```python
from build123d import *

# Parameters (mm, degrees)
SKETCH1_R                = 140
SKETCH1_R_2              = 97
BOSS_EXTRUDE1_DEPTH      = 112.5
SKETCH2_R                = 23.5
BOSS_EXTRUDE2_DEPTH      = 32
CIRPATTERN1_COUNT        = 3
MIRROR1_COPY_1_SKETCH_R  = 23.5
MIRROR1_COPY_1_DEPTH     = 32
MIRROR1_COPY_2_SKETCH_R  = 23.5
MIRROR1_COPY_2_DEPTH     = 32
SKETCH3_R                = 28.1
CUT_EXTRUDE1_DEPTH       = 310
BOSS_EXTRUDE3_REACH      = 450.894
BOSS_EXTRUDE3_END_RADIUS = 140
SKETCH4_R                = 100
SKETCH5_R                = 50
CUT_EXTRUDE2_DEPTH       = 25
SKETCH6_R                = 10.15
CUT_EXTRUDE3_DEPTH       = 13
BOSS_EXTRUDE4_REACH      = 400.629
BOSS_EXTRUDE4_END_RADIUS = 140
SKETCH7_R                = 37.5
SKETCH7_R_2              = 28.1
SKETCH8_R                = 37.5
BOSS_EXTRUDE5_DEPTH      = 10


with BuildPart() as part:
    # Sketch1 → Boss-Extrude1 (new, symmetric)
    with BuildSketch(Plane(origin=(0, 0, 0), x_dir=(1, 0, 0), z_dir=(0, 1, 0))):
        with Locations(Location((0, 0, 0), (0, 0, 270))):
            Circle(SKETCH1_R)
        with Locations(Location((0, 0, 0), (0, 0, 270))):
            Circle(SKETCH1_R_2, mode=Mode.SUBTRACT)
    extrude(amount=BOSS_EXTRUDE1_DEPTH, both=True)

    # Sketch2 → Boss-Extrude2 (add)
    with BuildSketch(Plane(origin=(0, 112.5, 0), x_dir=(1, 0, 0), z_dir=(0, 1, 0))):
        with BuildLine():
            ThreePointArc((175, -50), (225, 0), (175, 50))
            Line((175, 50), (130.766968306, 50))
            ThreePointArc((130.766968306, 50), (137.672392953, 25.42267135), (140, 0))
            ThreePointArc((140, 0), (137.672392953, -25.42267135), (130.766968306, -50))
            Line((130.766968306, -50), (175, -50))
        make_face()
        with Locations(Location((175, 0, 0), (0, 0, 270))):
            Circle(SKETCH2_R, mode=Mode.SUBTRACT)
    boss_extrude2 = extrude(amount=-BOSS_EXTRUDE2_DEPTH)

    # CirPattern1: Boss-Extrude2 ×3 about axis
    cirpattern1_axis = Axis((0, 0, 0), (0, 1, 0))
    for i in range(1, CIRPATTERN1_COUNT):
        add(boss_extrude2.rotate(cirpattern1_axis, i * 360 / CIRPATTERN1_COUNT))

    # Mirror1: Boss-Extrude2 across plane
    add(boss_extrude2.mirror(Plane.ZX))

    # Mirror1 copy 1 sketch → Mirror1 copy 1 (add)
    with BuildSketch(Plane(origin=(0, -112.5, 0), x_dir=(-0.4999999999999998, 0, -0.8660254037844387), z_dir=(0, -1, 0))):
        with BuildLine():
            ThreePointArc((175, 50), (225, 0), (175, -50))
            Line((175, -50), (130.766968306, -50))
            ThreePointArc((130.766968306, -50), (137.672392953, -25.42267135), (140, 0))
            ThreePointArc((140, 0), (137.672392953, 25.42267135), (130.766968306, 50))
            Line((130.766968306, 50), (175, 50))
        make_face()
        with Locations((175, 0)):
            Circle(MIRROR1_COPY_1_SKETCH_R, mode=Mode.SUBTRACT)
    extrude(amount=-MIRROR1_COPY_1_DEPTH)

    # Mirror1 copy 2 sketch → Mirror1 copy 2 (add)
    with BuildSketch(Plane(origin=(0, -112.5, 0), x_dir=(-0.5000000000000004, 0, 0.8660254037844384), z_dir=(0, -1, 0))):
        with BuildLine():
            ThreePointArc((175, 50), (225, 0), (175, -50))
            Line((175, -50), (130.766968306, -50))
            ThreePointArc((130.766968306, -50), (137.672392953, -25.42267135), (140, 0))
            ThreePointArc((140, 0), (137.672392953, 25.42267135), (130.766968306, 50))
            Line((130.766968306, 50), (175, 50))
        make_face()
        with Locations((175, 0)):
            Circle(MIRROR1_COPY_2_SKETCH_R, mode=Mode.SUBTRACT)
    extrude(amount=-MIRROR1_COPY_2_DEPTH)

    # Sketch3 → Cut-Extrude1 (cut)
    with BuildSketch(Plane(origin=(-160, 0, 0), x_dir=(0, 0, -1), z_dir=(1, 0, 0))):
        with Locations(Location((0, 0, 0), (0, 0, 180))):
            Circle(SKETCH3_R)
    extrude(amount=CUT_EXTRUDE1_DEPTH, mode=Mode.SUBTRACT)

    # Boss-Extrude3: up to this cylinder (the profile starts outside it)
    boss_extrude3_end = Plane(origin=(0, 0, 0), z_dir=(0, -1, 0)) * Cylinder(BOSS_EXTRUDE3_END_RADIUS, 1182.788, mode=Mode.PRIVATE)
    # Sketch4 → Boss-Extrude3 (add, up to the surface)
    with BuildSketch(Plane(origin=(-160, 0, 0), x_dir=(0, 0, -1), z_dir=(1, 0, 0)), mode=Mode.PRIVATE) as boss_extrude3_sk1:
        with Locations(Location((0, 0, 0), (0, 0, 180))):
            Circle(SKETCH4_R)
    boss_extrude3_tool1 = extrude(boss_extrude3_sk1.sketch, amount=BOSS_EXTRUDE3_REACH, mode=Mode.PRIVATE) - boss_extrude3_end
    add(boss_extrude3_tool1.solids().sort_by_distance((-160, 0, 0))[0])

    # Sketch5 → Cut-Extrude2 (cut)
    with BuildSketch(Plane.ZY.offset(160)):
        Circle(SKETCH5_R)
    extrude(amount=-CUT_EXTRUDE2_DEPTH, mode=Mode.SUBTRACT)

    # Sketch6 → Cut-Extrude3 (cut)
    with BuildSketch(Plane.ZY.offset(160)):
        with Locations((0, 75)):
            Circle(SKETCH6_R)
        with Locations((64.951905284, -37.5)):
            Circle(SKETCH6_R)
        with Locations((-64.951905284, -37.5)):
            Circle(SKETCH6_R)
    extrude(amount=-CUT_EXTRUDE3_DEPTH, mode=Mode.SUBTRACT)

    # Boss-Extrude4: up to this cylinder (the profile starts outside it)
    boss_extrude4_end = Plane(origin=(0, 0, 0), z_dir=(0, -1, 0)) * Cylinder(BOSS_EXTRUDE4_END_RADIUS, 1082.258, mode=Mode.PRIVATE)
    # Sketch7 → Boss-Extrude4 (add, up to the surface)
    with BuildSketch(Plane(origin=(165, 0, 0), x_dir=(0, 0, -1), z_dir=(1, 0, 0)), mode=Mode.PRIVATE) as boss_extrude4_sk1:
        Circle(SKETCH7_R)
        with Locations(Location((0, 0, 0), (0, 0, 180))):
            Circle(SKETCH7_R_2, mode=Mode.SUBTRACT)
    boss_extrude4_tool1 = extrude(boss_extrude4_sk1.sketch, amount=-BOSS_EXTRUDE4_REACH, mode=Mode.PRIVATE) - boss_extrude4_end
    add(boss_extrude4_tool1.solids().sort_by_distance((165, 0, 36.43934))[0])

    # Sketch8 → Boss-Extrude5 (add)
    with BuildSketch(Plane(origin=(165, 0, 0), x_dir=(0, 0, -1), z_dir=(1, 0, 0))):
        Circle(SKETCH8_R)
    extrude(amount=-BOSS_EXTRUDE5_DEPTH)


solid = part.part
```
Read the model definition and answer for the solid it produces. Units are mm, in the model's axes. A direction names the side the tool comes from. Coordinates: 2 decimals unless noted, no trailing zeros. Write each loop counter-clockwise with the first axis right and the second up, starting at its lowest first coordinate (ties: lowest second). Pieces come first, ordered by that corner, then holes. Notation, with made-up numbers: (83, 37.5) -> (124, 37.5) arc R26 ccw to (124, 73.5) -> close; hole circle Ø9 at (31.5, 73.5). An arc over 180 degrees is marked (long way). Answer as a JSON object with one key per item and string values.
Q1. The part is cut by section C-C on x = -87.5. Give the number of separate pieces and of enclosed holes in the cut face, then the cut area to 3 significant figures.
The answers:
{"separate pieces": "6", "enclosed holes": "0", "area": "36,100 mm2"}
Q2. The part is cut by section B-B on y = 75. Give the vertices of the cut face in (x, z).
The answers:
{"outline": "(-160, -66.14) -> (-123.39, -66.14) arc R140 ccw (long way) to (-123.39, 66.14) -> (-160, 66.14) -> (-160, 10.15) -> (-147, 10.15) -> (-147, -10.15) -> (-160, -10.15) -> close; hole circle Ø194 at (0, 0)"}
Q3. A tool of negligible diameter and unlimited length cuts with its end or side. For faces 1 (the cylindrical face through (198.3, 96.72, -3.06)), 2 (the cylindrical face through (198.3, -96.72, -3.06)), 3 (the cylindrical face through (-114.215, -1.236, -28.073)), 4 (the flat face through (153, -97, 50)), from which of +Z, -Z, +X, -X, +Y, -Y can it reach the whole face along a straight path? Write none if from no direction.
The answers:
{"face 1": "+Y", "face 2": "-Y", "face 3": "-X", "face 4": "+Z, +X, +Y, -Y"}
Q4. The part is cut by section A-A on x = 64.5. Give the vertices of the cut face in (y, z), then the cut area to 3 significant figures.
The answers:
{"outline": "(-112.5, -124.26) -> (112.5, -124.26) -> (112.5, -72.45) -> (-112.5, -72.45) -> close; (-112.5, 72.45) -> (112.5, 72.45) -> (112.5, 124.26) -> (-112.5, 124.26) -> close", "area": "23,300 mm2"}
Q5. Flat-ended cylindrical pins translate along their axes: pin 1 Ø1.5 at (x, y) = (62, 30) entering from -Z; pin 2 Ø8 at (x, y) = (-29, -32) entering from -Z; pin 3 Ø8 at (y, z) = (78, -132.5) entering from +X. Find the tip coordinate at first contact, or state that the pin passes through.
The answers:
{"pin 1": "stops at z = -125.89", "pin 2": "stops at z = -137.75", "pin 3": "stops at x = 55.57"}
Q6. Determine the mould class of faces 5 (the cylindrical face through (150.15, -14.36, -34.64)), 6 (the flat face through (97.4, -112.5, -0.9)), 7 (the flat face through (153, 97, -50)) for opening direction Y: pulls with the +Y half, pulls with the -Y half, needs draft (parallel to the pull), parting line crosses it, or undercut.
The answers:
{"face 5": "undercut", "face 6": "pulls with the -Y half", "face 7": "needs draft"}
Q7. The part is cut by section D-D on z = 149. Give the vertices of the cut face in (x, y), then the cut area to 3 significant figures.
The answers:
{"outline": "(-137.43, -112.5) -> (-110.86, -112.5) -> (-110.86, -80.5) -> (-137.43, -80.5) -> close; (-137.43, 80.5) -> (-110.86, 80.5) -> (-110.86, 112.5) -> (-137.43, 112.5) -> close; (-64.14, -112.5) -> (-28.29, -112.5) -> (-28.29, -80.5) -> (-64.14, -80.5) -> close; (-64.14, 80.5) -> (-28.29, 80.5) -> (-28.29, 112.5) -> (-64.14, 112.5) -> close", "area": "4,000 mm2"}
Q8. Consider line 1 (Y direction, x = -153, z = 0); line 2 (Y direction, x = 142, z = 0); line 3 (Y direction, x = 165.5, z = 47). Determine where each line is inside the solid, lowest interval first. Write a range as [from, to].
The answers:
{"line 1": "y = [-100, -50], [50, 64.85], [85.15, 100]", "line 2": "y = [-112.5, -80.5], [-37.5, -28.1], [28.1, 37.5], [80.5, 112.5]", "line 3": "y = [-112.5, -80.5], [80.5, 112.5]"}
